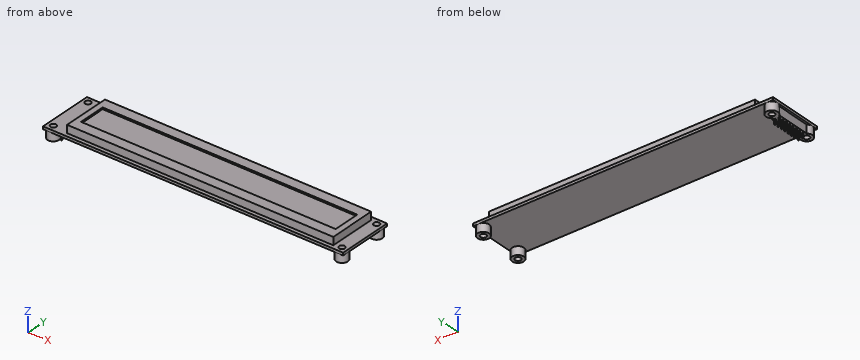
```python
from build123d import *

# Parameters (mm, degrees)
SKETCH_2_W                          = 182
SKETCH_2_H                          = 33.5
EXTRUDE_1_DEPTH                     = 1.6
SKETCH_3_W                          = 161.4
SKETCH_3_H                          = 28.9
EXTRUDE_2_DEPTH                     = 4.7
SKETCH_4_W                          = 154.4
SKETCH_4_H                          = 16.5
CUT_EXTRUDE_1_DEPTH                 = 1
SKETCH_6_R                          = 3.55
EXTRUDE_3_DEPTH                     = 5
SKETCH_5_R                          = 1.75
CUT_EXTRUDE_2_DEPTH                 = 93.821885889
SKETCH_7_W                          = 0.64
SKETCH_7_H                          = 0.64
EXTRUDE_4_DEPTH                     = 3.2
CHAMFER_1_SIZE                      = 0.2
CHAMFER_1_SIZE2                     = 0.307972993
SKETCH_9_W                          = 5
SKETCH_9_H                          = 20.32
EXTRUDE_5_DEPTH                     = 5
PATTERN_LINEAR_6_COUNT              = 8
PATTERN_LINEAR_6_PITCH              = 2.54
PATTERN_LINEAR_6_COUNT_DIR2         = 2
PATTERN_LINEAR_6_PITCH_DIR2         = 2.54
CHAMFER_1_OF_PATTERN_LINEAR_6_SIZE2 = 0.2
CHAMFER_1_OF_PATTERN_LINEAR_6_SIZE  = 0.307972993


with BuildPart() as part:
    # Sketch 2 → Extrude 1 (new body)
    with BuildSketch(Plane.XY.offset(5)):
        Rectangle(SKETCH_2_W, SKETCH_2_H)
    extrude(amount=EXTRUDE_1_DEPTH)

    # Sketch 3 → Extrude 2 (add)
    with BuildSketch(Plane.XY.offset(6.6)):
        with Locations((2.5, 0)):
            Rectangle(SKETCH_3_W, SKETCH_3_H)
    extrude(amount=EXTRUDE_2_DEPTH)

    # Sketch 4 → Cut-Extrude 1 (cut)
    with BuildSketch(Plane.XY.offset(11.3)):
        with Locations((2.5, 0)):
            Rectangle(SKETCH_4_W, SKETCH_4_H)
    extrude(amount=-CUT_EXTRUDE_1_DEPTH, mode=Mode.SUBTRACT)

    # Sketch 6 → Extrude 3 (add)
    with BuildSketch(Plane(origin=(0, 0, 5), x_dir=(-1, 0, 0), z_dir=(0, 0, -1))):
        with Locations(Location((-87.5, -13.25, 0), (0, 0, 189.627632683))):
            Circle(SKETCH_6_R)
        with Locations(Location((-87.5, 13.25, 0), (0, 0, 170.372367317))):
            Circle(SKETCH_6_R)
        with Locations(Location((87.5, 13.25, 0), (0, 0, 99.627632683))):
            Circle(SKETCH_6_R)
        with Locations(Location((87.5, -13.25, 0), (0, 0, 260.372367317))):
            Circle(SKETCH_6_R)
    extrude(amount=EXTRUDE_3_DEPTH)

    # Sketch 5 → Cut-Extrude 2 (cut, through all)
    with BuildSketch(Plane.XY.offset(6.6)):
        with Locations((-87.5, 13.25)):
            Circle(SKETCH_5_R)
        with Locations((-87.5, -13.25)):
            Circle(SKETCH_5_R)
        with Locations((87.5, -13.25)):
            Circle(SKETCH_5_R)
        with Locations((87.5, 13.25)):
            Circle(SKETCH_5_R)
    extrude(amount=-CUT_EXTRUDE_2_DEPTH, mode=Mode.SUBTRACT)



with BuildPart() as body_2:
    # Sketch 7 → Extrude 4 (new body)
    with BuildSketch(Plane.XY):
        with Locations((-88.5, -8.83)):
            Rectangle(SKETCH_7_W, SKETCH_7_H)
    extrude_4 = extrude(amount=-EXTRUDE_4_DEPTH)

    # Chamfer 1
    chamfer_1_edges = [body_2.edges().sort_by_distance(p)[0] for p in [
        (-88.18, -8.83, -3.2),
        (-88.5, -8.51, -3.2),
        (-88.82, -8.83, -3.2),
        (-88.5, -9.15, -3.2),
    ]]
    chamfer_1_side = [body_2.faces().sort_by_distance(p)[0] for p in [
        (-88.5, -8.83, -3.2),
    ]]
    chamfer(chamfer_1_edges, length=CHAMFER_1_SIZE, length2=CHAMFER_1_SIZE2, reference=chamfer_1_side[0])


with BuildPart() as part_1:
    add(part.part)

    add(body_2.part)  # Extrude 5 merges body 2
    # Sketch 9 → Extrude 5 (add)
    with BuildSketch(Plane.XY):
        with Locations((-87.23, 0)):
            Rectangle(SKETCH_9_W, SKETCH_9_H)
    extrude(amount=EXTRUDE_5_DEPTH)

    # Pattern Linear 6: Extrude 4 8 × 2
    with Locations(*[(j * PATTERN_LINEAR_6_PITCH_DIR2, i * PATTERN_LINEAR_6_PITCH, 0) for i in range(PATTERN_LINEAR_6_COUNT) for j in range(PATTERN_LINEAR_6_COUNT_DIR2) if (i, j) != (0, 0)]):
        add(extrude_4)

    # Chamfer 1 of Pattern Linear 6
    chamfer_1_of_pattern_linear_6_edges = [part_1.edges().sort_by_distance(p)[0] for p in [
        (-85.64, -8.83, -3.2),
        (-85.96, -8.51, -3.2),
        (-86.28, -8.83, -3.2),
        (-85.96, -9.15, -3.2),
        (-88.18, -6.29, -3.2),
        (-88.5, -5.97, -3.2),
        (-88.82, -6.29, -3.2),
        (-88.5, -6.61, -3.2),
        (-85.64, -6.29, -3.2),
        (-85.96, -5.97, -3.2),
        (-86.28, -6.29, -3.2),
        (-85.96, -6.61, -3.2),
        (-88.18, -3.75, -3.2),
        (-88.5, -3.43, -3.2),
        (-88.82, -3.75, -3.2),
        (-88.5, -4.07, -3.2),
        (-85.64, -3.75, -3.2),
        (-85.96, -3.43, -3.2),
        (-86.28, -3.75, -3.2),
        (-85.96, -4.07, -3.2),
        (-88.18, -1.21, -3.2),
        (-88.5, -0.89, -3.2),
        (-88.82, -1.21, -3.2),
        (-88.5, -1.53, -3.2),
        (-85.64, -1.21, -3.2),
        (-85.96, -0.89, -3.2),
        (-86.28, -1.21, -3.2),
        (-85.96, -1.53, -3.2),
        (-88.18, 1.33, -3.2),
        (-88.5, 1.65, -3.2),
        (-88.82, 1.33, -3.2),
        (-88.5, 1.01, -3.2),
        (-85.64, 1.33, -3.2),
        (-85.96, 1.65, -3.2),
        (-86.28, 1.33, -3.2),
        (-85.96, 1.01, -3.2),
        (-88.18, 3.87, -3.2),
        (-88.5, 4.19, -3.2),
        (-88.82, 3.87, -3.2),
        (-88.5, 3.55, -3.2),
        (-85.64, 3.87, -3.2),
        (-85.96, 4.19, -3.2),
        (-86.28, 3.87, -3.2),
        (-85.96, 3.55, -3.2),
        (-88.18, 6.41, -3.2),
        (-88.5, 6.73, -3.2),
        (-88.82, 6.41, -3.2),
        (-88.5, 6.09, -3.2),
        (-85.64, 6.41, -3.2),
        (-85.96, 6.73, -3.2),
        (-86.28, 6.41, -3.2),
        (-85.96, 6.09, -3.2),
        (-88.18, 8.95, -3.2),
        (-88.5, 9.27, -3.2),
        (-88.82, 8.95, -3.2),
        (-88.5, 8.63, -3.2),
        (-85.64, 8.95, -3.2),
        (-85.96, 9.27, -3.2),
        (-86.28, 8.95, -3.2),
        (-85.96, 8.63, -3.2),
    ]]
    chamfer(chamfer_1_of_pattern_linear_6_edges, length=CHAMFER_1_OF_PATTERN_LINEAR_6_SIZE, length2=CHAMFER_1_OF_PATTERN_LINEAR_6_SIZE2)


solid = part_1.part
```
The listing builds one solid part. Answer for the finished solid, in the listing's coordinates (mm). Round coordinates to 2 decimals unless told otherwise and drop trailing zeros. Loops run counter-clockwise (first coordinate to the right, second up) from the corner with the lowest first, then second, coordinate; pieces in that order, holes last.
1) Given P1, Ø2.5, axis at x = 13.5, z = 8, coming from the +Y side; P2, Ø1, axis at x = -51.5, z = 4, coming from the -Y side; P3, Ø1.5, axis at x = 58.5, y = 5.5, coming from the +Z side; P4, Ø0.7, axis at y = 6.5, z = -1.5, coming from the +X side, each flat-ended and moving along its own axis, determine where each tip first touches the part or whether it passes through.
Outcome:
P1: stops at y = 14.45
P2: passes through
P3: stops at z = 10.3
P4: stops at x = -85.64
2) A cutting plane is placed at A-A on x = 21.5. Determine the outline of the cut face in (y, z), plus the area to 3 significant figures.
Outcome:
outline: (-16.75, 5) - (16.75, 5) - (16.75, 6.6) - (14.45, 6.6) - (14.45, 11.3) - (8.25, 11.3) - (8.25, 10.3) - (-8.25, 10.3) - (-8.25, 11.3) - (-14.45, 11.3) - (-14.45, 6.6) - (-16.75, 6.6) - close
area: 173 mm2
3) Consider line 1 (Y direction, x = 87.5, z = 1.5); line 2 (Y direction, x = -87.5, z = 4); line 3 (Z direction, x = 45, y = 4). Determine where each line is inside the solid, lowest interval first.
Outcome:
line 1: y = -16.8 to -15, -11.5 to -9.7, 9.7 to 11.5, 15 to 16.8
line 2: y = -16.8 to -15, -11.5 to 11.5, 15 to 16.8
line 3: z = 5 to 10.3
